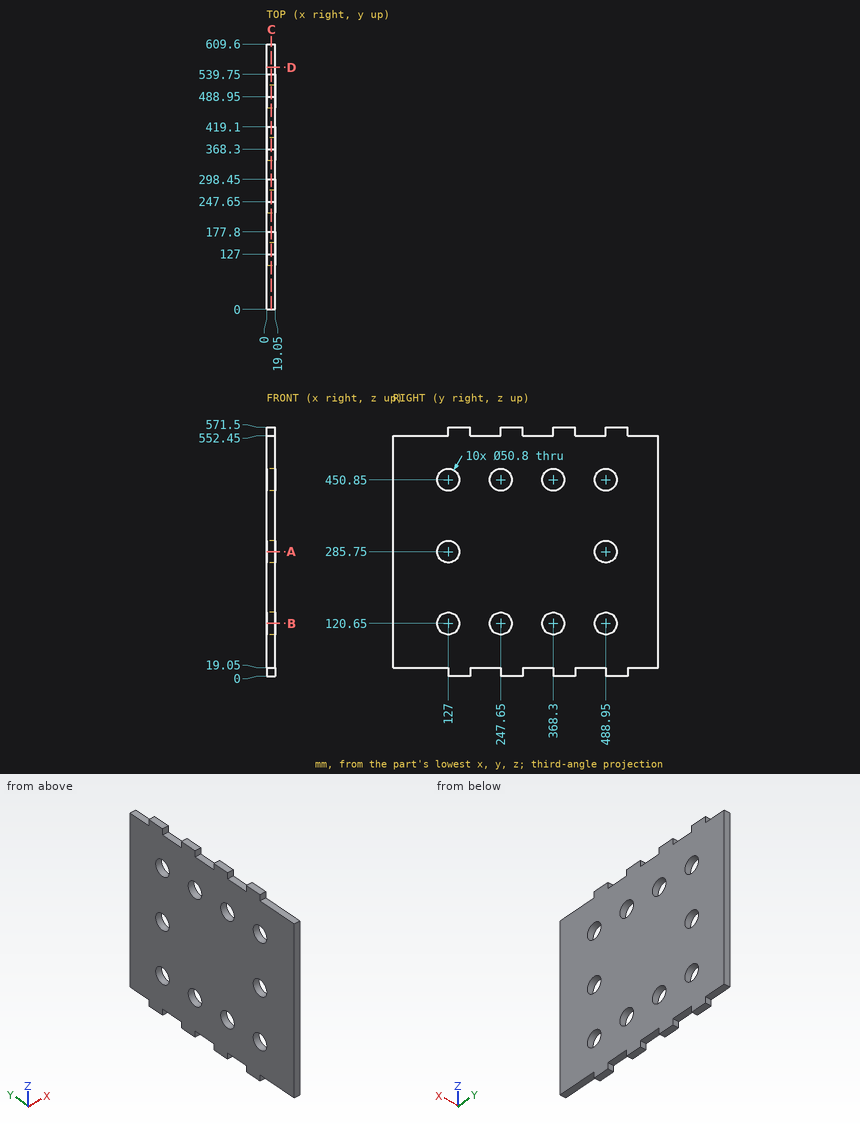
Drawing for the job (mm, zero at the part's lowest x, y, z). Coordinates: 2 decimals unless noted, no trailing zeros. Order: outer loops, then holes, each group sorted by start corner. A loop starts at its lowest first (then second) coordinate and runs counter-clockwise, first axis right, second up. Notation, with made-up numbers: (-36, 75.5) - (-25, 75.5) arc R24 cw to (-25, 100.5) - close; hole circle Ø7 at (47, -5). An arc over 180 degrees is marked (long way). Use a Markdown table: item, result. Add a question column.
(1) Saw through at A-A (z = 285.75). Give the cut face in (x, y), then the cut area to 3 significant figures.
(2) Saw through at B-B (z = 120.65). Give the cut face in (x, y), then the cut area to 3 significant figures.
(3) Saw through at D-D (y = 556). Give the cut face in (x, z).
(4) Drill centre lines: line 1 along Y through (x, z) = (14, 451.5); line 2 along Z through (x, y) = (5, 121.5); line 3 along Y through (x, z) = (5, 273.5). Where is each one in solid material? Low to high. Write a range as [from, to].
(5) Flat gauge pins, fed straight in: pin 1 (5 mm diameter, centred on x = 6.5, z = 263.5, fed in from -Y); pin 2 (9.5 mm diameter, centred on x = 9.5, z = 559, fed in from -Y); pin 3 (5.5 mm diameter, centred on x = 11.5, y = 341, fed in from -Z); pin 4 (9.5 mm diameter, centred on x = 10.5, z = 558, fed in from +Y). Where does each tip first touch, or does it go through?
(6) Saw through at C-C (x = 11). Count the separate pieces of the cut face and the enclosed holes in it, then the cut area to 3 significant figures.
Solved:
| question | item | result |
|---|---|---|
| 1 | outline | (0, 0) - (19.05, 0) - (19.05, 101.6) - (0, 101.6) - close; (0, 152.4) - (19.05, 152.4) - (19.05, 463.55) - (0, 463.55) - close; (0, 514.35) - (19.05, 514.35) - (19.05, 609.6) - (0, 609.6) - close |
| 1 | area | 9,680 mm² |
| 2 | outline | (0, 0) - (19.05, 0) - (19.05, 101.6) - (0, 101.6) - close; (0, 152.4) - (19.05, 152.4) - (19.05, 222.25) - (0, 222.25) - close; (0, 273.05) - (19.05, 273.05) - (19.05, 342.9) - (0, 342.9) - close; (0, 393.7) - (19.05, 393.7) - (19.05, 463.55) - (0, 463.55) - close; (0, 514.35) - (19.05, 514.35) - (19.05, 609.6) - (0, 609.6) - close |
| 2 | area | 7,740 mm² |
| 3 | outline | (0, 19.05) - (19.05, 19.05) - (19.05, 552.45) - (0, 552.45) - close |
| 4 | line 1 | y = [0, 101.61], [152.39, 222.26], [273.04, 342.91], [393.69, 463.56], [514.34, 609.6] |
| 4 | line 2 | z = [19.05, 95.85], [145.45, 260.95], [310.55, 426.05], [475.65, 552.45] |
| 4 | line 3 | y = [0, 104.75], [149.25, 466.7], [511.2, 609.6] |
| 5 | pin 1 | stops at y = 0 |
| 5 | pin 2 | stops at y = 127 |
| 5 | pin 3 | stops at z = 19.05 |
| 5 | pin 4 | stops at y = 539.75 |
| 6 | separate pieces | 1 |
| 6 | enclosed holes | 10 |
| 6 | area | 313,000 mm² |
